Autodesk Inventor part; units mm, degrees
ref_plane "YZ Plane" through (0, 0, 0) normal (1, 0, 0) x (0, 1, 0)
ref_plane "XZ Plane" through (0, 0, 0) normal (0, 1, 0) x (-1, 0, 0)
ref_plane "XY Plane" through (0, 0, 0) normal (0, 0, 1) x (1, 0, 0)
sketch "スケッチ1" plane through (0, 0, 0) normal (0, 0, 1) x (1, 0, 0)
  circle A0 centre (0, 0) radius 7.5
  circle A1 centre (0, 0) radius 30
  circle A2 centre (0, 0) radius 37.5
  circle A3 centre (23.5425, -29.1891) radius 30
  circle A4 centre (23.5425, -29.1891) radius 4
  circle A5 centre (23.5425, -29.1891) radius 16
  circle A6 centre (23.5425, -29.1891) radius 56
  circle A7 centre (0, -80) radius 40
  circle A8 centre (0, -80) radius 50
  circle A9 centre (0, -80) radius 4
  dimension "d57" = 75
  dimension "d64" = 112
  dimension "d41" = 15
  dimension "d58" = 8
  dimension "d63" = 32
  dimension "d65" = 100
  dimension "d66" = 8
sketch "スケッチ2" plane through (0, 0, 0) normal (0, 0, 1) x (1, 0, 0)
  line L0 (0, 0) -> (24.502, 0) construction
  line L1 (0, 0) -> (12.5, 0) construction
  line L2 (0, 0) -> (10.253, 10.253)
  line L3 (0, 0) -> (14.5, 0) construction
  line L4 (10.253, 10.253) -> (-10.253, -10.253)
  circle A0 centre (10.253, 10.253) radius 2
  circle A1 centre (-10.253, -10.253) radius 2
  circle A2 centre (0, 0) radius 7.5
  line L5 (0, 0) -> (28.1908, 10.2606)
  line L6 (0, 0) -> (30, 0) construction
  line L7 (0, 0) -> (-28.1908, 10.2606)
  line L8 (0, 0) -> (30, 0) construction
  circle A3 centre (-28.1908, 10.2606) radius 2.5
  line L9 (0, 0) -> (0, 30)
  circle A4 centre (0, 30) radius 2.5
  circle A5 centre (28.1908, 10.2606) radius 2.5
  dimension "d9" = 14.5
  dimension "d10" = 45
  dimension "d11" = 29
  dimension "d12" = 4
  dimension "d13" = 4
  dimension "d14" = 15
  dimension "d15" = 30
  dimension "d16" = 20
  dimension "d17" = 30
  dimension "d18" = 160
  dimension "d19" = 5
  dimension "d20" = 30
  dimension "d21" = 5
  dimension "d22" = 5
sketch "スケッチ3" plane through (0, 0, 0) normal (0, 0, 1) x (1, 0, 0)
  line L0 (60, -99.3436) -> (-60, -99.3436)
  line L1 (-60, -99.3436) -> (-60, 99.3436)
  line L2 (-60, 99.3436) -> (60, 99.3436)
  line L3 (60, 99.3436) -> (60, -99.3436)
  line L4 (60, -99.3436) -> (-60, 99.3436) construction
  line L5 (-60, -99.3436) -> (60, 99.3436) construction
  point P0 (0, 0)
  dimension "d25" = 120
extrude "押し出し1" add sketch "スケッチ3" against normal blind 3
sketch "スケッチ4" plane through (0, 0, 0) normal (0, 0, 1) x (1, 0, 0)
  line L0 (0, 45.0711) -> (68.3595, 45.0711)
  line L1 (68.3595, 45.0711) -> (-74.3824, 45.0711)
  line L2 (-74.3824, 45.0711) -> (108.1656, 45.0711)
  line L3 (108.1656, 45.0711) -> (108.1656, 129.4154)
  line L4 (108.1656, 129.4154) -> (-74.3824, 129.4154)
  line L5 (-74.3824, 129.4154) -> (-74.3824, 45.0711)
  point P0 (0, 0)
extrude "押し出し4" cut sketch "スケッチ4" against normal blind 10
fillet "フィレット1" radius 4 4 edges at (-60, 45.0711, -1.5) (60, 45.0711, -1.5) (-60, -99.3436, -1.5) (60, -99.3436, -1.5)
extrude "押し出し9" cut sketch "スケッチ1" against normal blind 10 contours A4 A2 | A2 A4 | A9 A6 | A6 A9
sketch "スケッチ8" plane through (0, 0, 0) normal (0, 0, 1) x (1, 0, 0)
  line L0 (-265.6992, -158.784) -> (100.3409, -158.784)
  line L1 (100.3409, -158.784) -> (100.3409, -94)
  line L2 (100.3409, -94) -> (-265.6992, -94)
  line L3 (-265.6992, -94) -> (-265.6992, -158.784)
  line L4 (-265.6992, -158.784) -> (100.3409, -94) construction
  line L5 (100.3409, -158.784) -> (-265.6992, -94) construction
  point P0 (0, 0)
  point P1 (0, -94)
  point P2 (-82.6791, -126.392)
extrude "押し出し10" cut sketch "スケッチ8" against normal blind 10
extrude "押し出し11" cut sketch "スケッチ2" against normal blind 10 contours A0 | A5 | A1 | A3 | A4
sketch "スケッチ9" plane through (0, 0, -3) normal (0, 0, -1) x (-1, 0, 0)
  line L0 (60, -94) -> (-60, -94)
  circle A0 centre (-50, -84) radius 2
  circle A1 centre (-50, -70) radius 2
  circle A2 centre (50, -70) radius 2
  circle A3 centre (50, -84) radius 2
  point P0 (0, 0)
  point P1 (-50, -94)
  point P2 (50, -94)
  dimension "d73" = 4
  dimension "d74" = 4
  dimension "d75" = 4
  dimension "d76" = 4
extrude "押し出し12" cut sketch "スケッチ9" against normal blind 10
sketch "スケッチ10" plane through (0, 0, 0) normal (0, 0, 1) x (1, 0, 0)
  circle A0 centre (23.5425, -29.1891) radius 4
  circle A1 centre (23.5425, -29.1891) radius 11
  circle A2 centre (0, -80) radius 4
  circle A3 centre (0, -80) radius 11
  point P0 (0, 0)
  dimension "d79" = 22
  dimension "d80" = 22
extrude "押し出し13" cut sketch "スケッチ10" against normal blind 10
properties part number "板" material "アルミニウム 6061"
Design review of the part built by this model. Coordinates are the model's own, in mm. Give positions to 0.01 mm unless a question says otherwise; leave off trailing zeros. Write each loop counter-clockwise with the first axis right and the second up, starting at its lowest first coordinate (ties: lowest second). Pieces come first, ordered by that corner, then holes. Notation, with made-up numbers: (1, 37) -> (50, 37) arc R26 ccw to (50, 60) -> close; hole circle Ø2 at (-29, 65.5). An arc over 180 degrees is marked (long way). Answer in a Markdown table with one row per item.
(1) Consider section A-A (x = 0). State the section outline as (y, z) points.
Results:
| item | result |
|---|---|
| outline | (-94, -3) -> (-91, -3) -> (-91, 0) -> (-94, 0) -> close; (-69, -3) -> (27.5, -3) -> (27.5, 0) -> (-69, 0) -> close; (32.5, -3) -> (45.07, -3) -> (45.07, 0) -> (32.5, 0) -> close |
(2) To check wall thickness, follow probe 1 along Y at (x, z) = (50, -1.05); probe 2 along Y at (x, z) = (49.5, -1.4); probe 3 along Y at (x, z) = (25.5, -2.4). State the ranges of each line that lie inside material, in increasing order.
Results:
| item | result |
|---|---|
| probe 1 | -94 to -86, -82 to -72, -68 to 45.07 |
| probe 2 | -94 to -85.94, -82.06 to -71.94, -68.06 to 45.07 |
| probe 3 | -94 to -40.01, -18.36 to 45.07 |
(3) Consider section C-C (z = -1.1). Count the separate pieces of the cut face and the enclosed holes in it, then the cut area to 3 significant figures.
Results:
| item | result |
|---|---|
| separate pieces | 1 |
| enclosed holes | 11 |
| area | 15,800 mm2 |
(4) Consider section B-B (y = 30). State the section outline as (x, z) points, then the cut area to 3 significant figures.
Results:
| item | result |
|---|---|
| outline | (-60, -3) -> (-2.5, -3) -> (-2.5, 0) -> (-60, 0) -> close; (2.5, -3) -> (60, -3) -> (60, 0) -> (2.5, 0) -> close |
| area | 345 mm2 |
(5) Consider section D-D (y = -84). State the section outline as (x, z) points.
Results:
| item | result |
|---|---|
| outline | (-60, -3) -> (-52, -3) -> (-52, 0) -> (-60, 0) -> close; (-48, -3) -> (-10.25, -3) -> (-10.25, 0) -> (-48, 0) -> close; (10.25, -3) -> (48, -3) -> (48, 0) -> (10.25, 0) -> close; (52, -3) -> (60, -3) -> (60, 0) -> (52, 0) -> close |
(6) Mouldability with a two-part tool opening along Y and no side actions: class faces 1 (the cylindrical face through (58.86, 43.87, -1.48)), 2 (the cylindrical face through (26.207, 8.739, -1.479)), 3 (the flat face through (-1, -23, 0)) as +Y half, -Y half, draft (parallel to the pull), parting line (faces both ways), or undercut.
Results:
| item | result |
|---|---|
| face 1 | +Y half |
| face 2 | undercut |
| face 3 | draft |
(7) Clearance check with a flat-ended pin moving along its axis: pin 1 (2.5 mm diameter, centred on x = -50, y = -84, fed in from -Z) (3 decimals). State where the tip first meets the part, or that it passes through.
Results:
| item | result |
|---|---|
| pin 1 | through |
